Geometry check sheet. Reference: the model listing, model coordinates, mm. A direction names the side the tool comes from. Round coordinates to 2 decimals unless told otherwise and drop trailing zeros. Write each loop counter-clockwise with the first axis right and the second up, starting at its lowest first coordinate (ties: lowest second). Pieces come first, ordered by that corner, then holes. Notation, with made-up numbers: (64, 37) -> (111, 37) arc R24 ccw to (111, 73) -> close; hole circle Ø6 at (-6.75, -11). An arc over 180 degrees is marked (long way). Use a Markdown table: item, result.
```python
from build123d import *

# Parameters (mm, degrees)
F0_R     = 6.35
F1_DEPTH = 5.08


with BuildPart() as f1:
    # F0 (on Top) → F1 (new body)
    with BuildSketch(Plane.XY):
        with BuildLine():
            Line((-4.392071, 95.772413), (-4.392071, 85.612413))
            ThreePointArc((-4.392071, 85.612413), (-8.960703, 85.255389), (-13.503728, 84.65474))
            Line((-13.503728, 84.65474), (-15.616111, 94.592719))
            ThreePointArc((-15.616111, 94.592719), (-20.252225, 95.279225), (-24.208298, 92.766394))
            Line((-24.208298, 92.766394), (-22.095915, 82.828414))
            ThreePointArc((-22.095915, 82.828414), (-26.490482, 81.52932), (-30.80935, 79.997247))
            Line((-30.80935, 79.997247), (-34.941794, 89.278869))
            ThreePointArc((-34.941794, 89.278869), (-39.61933, 88.986471), (-42.966506, 85.706037))
            Line((-42.966506, 85.706037), (-38.834062, 76.424415))
            ThreePointArc((-38.834062, 76.424415), (-42.8625, 74.240028), (-46.768454, 71.843492))
            Line((-46.768454, 71.843492), (-52.740352, 80.063104))
            ThreePointArc((-52.740352, 80.063104), (-57.25488, 78.804582), (-59.846872, 74.899916))
            Line((-59.846872, 74.899916), (-53.874974, 66.680303))
            ThreePointArc((-53.874974, 66.680303), (-57.361221, 63.70609), (-60.683553, 60.549831))
            Line((-60.683553, 60.549831), (-68.233905, 67.348198))
            ThreePointArc((-68.233905, 67.348198), (-72.388117, 65.178554), (-74.111642, 60.820309))
            Line((-74.111642, 60.820309), (-66.561291, 54.021942))
            ThreePointArc((-66.561291, 54.021942), (-69.352982, 50.387891), (-71.94649, 46.609851))
            Line((-71.94649, 46.609851), (-80.745308, 51.689851))
            ThreePointArc((-80.745308, 51.689851), (-84.357647, 48.70391), (-85.137378, 44.082562))
            Line((-85.137378, 44.082562), (-76.33856, 39.002562))
            ThreePointArc((-76.33856, 39.002562), (-78.313684, 34.867499), (-80.065019, 30.632798))
            Line((-80.065019, 30.632798), (-89.727753, 33.772411))
            ThreePointArc((-89.727753, 33.772411), (-92.640342, 30.100672), (-92.442202, 25.418196))
            Line((-92.442202, 25.418196), (-82.779468, 22.278583))
            ThreePointArc((-82.779468, 22.278583), (-83.851703, 17.82323), (-84.684323, 13.316944))
            Line((-84.684323, 13.316944), (-94.788666, 14.378954))
            ThreePointArc((-94.788666, 14.378954), (-96.87421, 10.18189), (-95.706859, 5.642933))
            Line((-95.706859, 5.642933), (-85.602516, 4.580924))
            ThreePointArc((-85.602516, 4.580924), (-85.725, 0), (-85.602516, -4.580924))
            Line((-85.602516, -4.580924), (-95.706859, -5.642933))
            ThreePointArc((-95.706859, -5.642933), (-96.87421, -10.18189), (-94.788666, -14.378954))
            Line((-94.788666, -14.378954), (-84.684323, -13.316944))
            ThreePointArc((-84.684323, -13.316944), (-83.851703, -17.82323), (-82.779468, -22.278583))
            Line((-82.779468, -22.278583), (-92.442202, -25.418196))
            ThreePointArc((-92.442202, -25.418196), (-92.640342, -30.100672), (-89.727753, -33.772411))
            Line((-89.727753, -33.772411), (-80.065019, -30.632798))
            ThreePointArc((-80.065019, -30.632798), (-78.313684, -34.867499), (-76.33856, -39.002562))
            Line((-76.33856, -39.002562), (-85.137378, -44.082562))
            ThreePointArc((-85.137378, -44.082562), (-84.357647, -48.70391), (-80.745308, -51.689851))
            Line((-80.745308, -51.689851), (-71.94649, -46.609851))
            ThreePointArc((-71.94649, -46.609851), (-69.352982, -50.387891), (-66.561291, -54.021942))
            Line((-66.561291, -54.021942), (-74.111642, -60.820309))
            ThreePointArc((-74.111642, -60.820309), (-72.388117, -65.178554), (-68.233905, -67.348198))
            Line((-68.233905, -67.348198), (-60.683553, -60.549831))
            ThreePointArc((-60.683553, -60.549831), (-57.361221, -63.70609), (-53.874974, -66.680303))
            Line((-53.874974, -66.680303), (-59.846872, -74.899916))
            ThreePointArc((-59.846872, -74.899916), (-57.25488, -78.804582), (-52.740352, -80.063104))
            Line((-52.740352, -80.063104), (-46.768454, -71.843492))
            ThreePointArc((-46.768454, -71.843492), (-42.8625, -74.240028), (-38.834062, -76.424415))
            Line((-38.834062, -76.424415), (-42.966506, -85.706037))
            ThreePointArc((-42.966506, -85.706037), (-39.61933, -88.986471), (-34.941794, -89.278869))
            Line((-34.941794, -89.278869), (-30.80935, -79.997247))
            ThreePointArc((-30.80935, -79.997247), (-26.490482, -81.52932), (-22.095915, -82.828414))
            Line((-22.095915, -82.828414), (-24.208298, -92.766394))
            ThreePointArc((-24.208298, -92.766394), (-20.252225, -95.279225), (-15.616111, -94.592719))
            Line((-15.616111, -94.592719), (-13.503728, -84.65474))
            ThreePointArc((-13.503728, -84.65474), (-8.960703, -85.255389), (-4.392071, -85.612413))
            Line((-4.392071, -85.612413), (-4.392071, -95.772413))
            ThreePointArc((-4.392071, -95.772413), (0, -97.40782), (4.392071, -95.772413))
            Line((4.392071, -95.772413), (4.392071, -85.612413))
            ThreePointArc((4.392071, -85.612413), (8.960703, -85.255389), (13.503728, -84.65474))
            Line((13.503728, -84.65474), (15.616111, -94.592719))
            ThreePointArc((15.616111, -94.592719), (20.252225, -95.279225), (24.208298, -92.766394))
            Line((24.208298, -92.766394), (22.095915, -82.828414))
            ThreePointArc((22.095915, -82.828414), (26.490482, -81.52932), (30.80935, -79.997247))
            Line((30.80935, -79.997247), (34.941794, -89.278869))
            ThreePointArc((34.941794, -89.278869), (39.61933, -88.986471), (42.966506, -85.706037))
            Line((42.966506, -85.706037), (38.834062, -76.424415))
            ThreePointArc((38.834062, -76.424415), (42.8625, -74.240028), (46.768454, -71.843492))
            Line((46.768454, -71.843492), (52.740352, -80.063104))
            ThreePointArc((52.740352, -80.063104), (57.25488, -78.804582), (59.846872, -74.899916))
            Line((59.846872, -74.899916), (53.874974, -66.680303))
            ThreePointArc((53.874974, -66.680303), (57.361221, -63.70609), (60.683553, -60.549831))
            Line((60.683553, -60.549831), (68.233905, -67.348198))
            ThreePointArc((68.233905, -67.348198), (72.388117, -65.178554), (74.111642, -60.820309))
            Line((74.111642, -60.820309), (66.561291, -54.021942))
            ThreePointArc((66.561291, -54.021942), (69.352982, -50.387891), (71.94649, -46.609851))
            Line((71.94649, -46.609851), (80.745308, -51.689851))
            ThreePointArc((80.745308, -51.689851), (84.357647, -48.70391), (85.137378, -44.082562))
            Line((85.137378, -44.082562), (76.33856, -39.002562))
            ThreePointArc((76.33856, -39.002562), (78.313684, -34.867499), (80.065019, -30.632798))
            Line((80.065019, -30.632798), (89.727753, -33.772411))
            ThreePointArc((89.727753, -33.772411), (92.640342, -30.100672), (92.442202, -25.418196))
            Line((92.442202, -25.418196), (82.779468, -22.278583))
            ThreePointArc((82.779468, -22.278583), (83.851703, -17.82323), (84.684323, -13.316944))
            Line((84.684323, -13.316944), (94.788666, -14.378954))
            ThreePointArc((94.788666, -14.378954), (96.87421, -10.18189), (95.706859, -5.642933))
            Line((95.706859, -5.642933), (85.602516, -4.580924))
            ThreePointArc((85.602516, -4.580924), (85.725, 0), (85.602516, 4.580924))
            Line((85.602516, 4.580924), (95.706859, 5.642933))
            ThreePointArc((95.706859, 5.642933), (96.87421, 10.18189), (94.788666, 14.378954))
            Line((94.788666, 14.378954), (84.684323, 13.316944))
            ThreePointArc((84.684323, 13.316944), (83.851703, 17.82323), (82.779468, 22.278583))
            Line((82.779468, 22.278583), (92.442202, 25.418196))
            ThreePointArc((92.442202, 25.418196), (92.640342, 30.100672), (89.727753, 33.772411))
            Line((89.727753, 33.772411), (80.065019, 30.632798))
            ThreePointArc((80.065019, 30.632798), (78.313684, 34.867499), (76.33856, 39.002562))
            Line((76.33856, 39.002562), (85.137378, 44.082562))
            ThreePointArc((85.137378, 44.082562), (84.357647, 48.70391), (80.745308, 51.689851))
            Line((80.745308, 51.689851), (71.94649, 46.609851))
            ThreePointArc((71.94649, 46.609851), (69.352982, 50.387891), (66.561291, 54.021942))
            Line((66.561291, 54.021942), (74.111642, 60.820309))
            ThreePointArc((74.111642, 60.820309), (72.388117, 65.178554), (68.233905, 67.348198))
            Line((68.233905, 67.348198), (60.683553, 60.549831))
            ThreePointArc((60.683553, 60.549831), (57.361221, 63.70609), (53.874974, 66.680303))
            Line((53.874974, 66.680303), (59.846872, 74.899916))
            ThreePointArc((59.846872, 74.899916), (57.25488, 78.804582), (52.740352, 80.063104))
            Line((52.740352, 80.063104), (46.768454, 71.843492))
            ThreePointArc((46.768454, 71.843492), (42.8625, 74.240028), (38.834062, 76.424415))
            Line((38.834062, 76.424415), (42.966506, 85.706037))
            ThreePointArc((42.966506, 85.706037), (39.61933, 88.986471), (34.941794, 89.278869))
            Line((34.941794, 89.278869), (30.80935, 79.997247))
            ThreePointArc((30.80935, 79.997247), (26.490482, 81.52932), (22.095915, 82.828414))
            Line((22.095915, 82.828414), (24.208298, 92.766394))
            ThreePointArc((24.208298, 92.766394), (20.252225, 95.279225), (15.616111, 94.592719))
            Line((15.616111, 94.592719), (13.503728, 84.65474))
            ThreePointArc((13.503728, 84.65474), (8.960703, 85.255389), (4.392071, 85.612413))
            Line((4.392071, 85.612413), (4.392071, 95.772413))
            ThreePointArc((4.392071, 95.772413), (0, 97.40782), (-4.392071, 95.772413))
        make_face()
        Circle(F0_R, mode=Mode.SUBTRACT)
    extrude(amount=F1_DEPTH)


solid = f1.part
```
(1) Section check B-B on y = 0. Record the cut outline in (x, z) (3 decimals).
A:
| item | result |
|---|---|
| outline | (-85.725, 0) -> (-6.35, 0) -> (-6.35, 5.08) -> (-85.725, 5.08) -> close; (6.35, 0) -> (85.725, 0) -> (85.725, 5.08) -> (6.35, 5.08) -> close |
(2) Gauge pin test, flat ends, axial feed: pin 1 Ø10 at (x, y) = (0, 0) entering from +Z; pin 2 Ø2 at (y, z) = (-70.5, 1.5) entering from +X; pin 3 Ø2 at (x, z) = (56, 2.5) entering from -Y; pin 4 Ø1.5 at (y, z) = (-92, 2.5) entering from -X. Record the tip position at first contact, or that the pin passes through.
A:
| item | result |
|---|---|
| pin 1 | passes through |
| pin 2 | stops at x = 57.38 |
| pin 3 | stops at y = -79.87 |
| pin 4 | stops at x = -24.2 |
(3) Access from +Z, -Z, +X, -X, +Y, -Y to the whole of each face (thin tool, end or side, straight path). Record for faces 1 (the face through (4.392, -91, 3)), 2 (the face through (90.584, 5.104, 2.504)), 3 (the face through (-89.807, -13.855, 2.504)), 4 (the face through (-80.8, 41.58, 2.5)).
A:
| item | result |
|---|---|
| face 1 | +Z, -Z, -Y |
| face 2 | +Z, -Z, +X |
| face 3 | +Z, -Z |
| face 4 | +Z, -Z, -X |
(4) Thickness scan on line 1 (Y direction, x = 73.5, z = 1.1); line 2 (X direction, y = -4, z = 2.65); line 3 (Y direction, x = -3.5, z = 1.35). Record the ranges inside material, lowest first.
A:
| item | result |
|---|---|
| line 1 | y = -63.49 to -60.27, -47.51 to 47.51, 60.27 to 63.49 |
| line 2 | x = -85.63 to -4.93, 4.93 to 85.63 |
| line 3 | y = -96.42 to -5.3, 5.3 to 96.42 |
(5) Section check A-A on x = 0. Record the cut outline in (y, z), plus the area to 3 significant figures.
A:
| item | result |
|---|---|
| outline | (-97.41, 0) -> (-6.35, 0) -> (-6.35, 5.08) -> (-97.41, 5.08) -> close; (6.35, 0) -> (97.41, 0) -> (97.41, 5.08) -> (6.35, 5.08) -> close |
| area | 925 mm2 |
